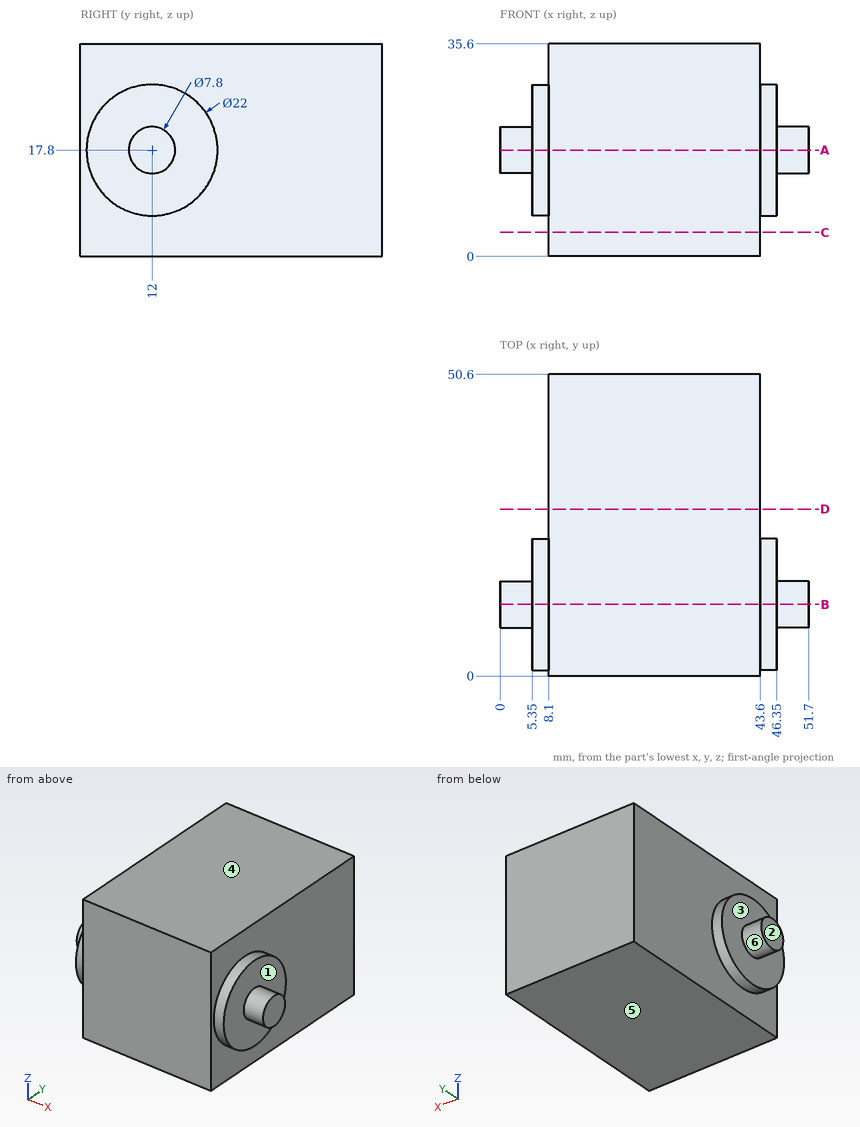
The figure shows three views and two pictorial views of one solid part (mm, origin at its lowest corner). Answer the questions. A direction names the side the tool comes from. Give positions to 0.01 mm unless a question says otherwise; leave off trailing zeros. Loops run counter-clockwise (first coordinate to the right, second up) from the corner with the lowest first, then second, coordinate; pieces in that order, holes last. Notation, with made-up numbers: (-3, 63) -> (56, 63) arc R28 ccw to (56, 85) -> close; hole circle Ø2 at (44, 25). An arc over 180 degrees is marked (long way). Put each result on its own line as item: value. Start each with the question number.
Item 1: Which of the six approach directions +Z, -Z, +X, -X, +Y, -Y give full straight-line access (tool end or side, diameter ignored) to the marked faces 1 and 2?
Item 2: Find the intervals of material crossed by L1, parallel to X at y = 46, z = 6; L2, parallel to X at y = 11, z = 9.5, in increasing order. Write a range as [from, to].
Item 3: The mould has two halves that part along Z. Classify the marked faces 3, 4, 5 and 6: released by +Z, released by -Z, zero draft, split by the parting line, or undercut.
Item 4: The part is cut by section C-C (z = 4). Give the vertices of the cut face in (x, y).
Item 5: The part is cut by section D-D (y = 28). Give the vertices of the cut face in (x, z).
Item 6: The part is cut by section A-A (z = 17.8). Give the vertices of the cut face in (x, y).
Item 7: The part is cut by section B-B (y = 12). Give the vertices of the cut face in (x, z).
Item 8: Each of these flat-tipped pins is pushed along its axis until it touches: P1, Ø2, axis at x = 38, z = 17.5, coming from the -Y side; P2, Ø1.5, axis at y = 35.5, z = 30, coming from the +X side; P3, Ø10, axis at y = 6.5, z = 27.5, coming from the -X side. Where does it stop, or does it pass through?
Answers below:
1. face 1: +X
1. face 2: +Z, -Z, -X, +Y, -Y
2. L1: [8.1, 43.6]
2. L2: [5.35, 46.35]
3. face 3: zero draft
3. face 4: released by +Z
3. face 5: released by -Z
3. face 6: split by the parting line
4. outline: (8.1, 0) -> (43.6, 0) -> (43.6, 50.6) -> (8.1, 50.6) -> close
5. outline: (8.1, 0) -> (43.6, 0) -> (43.6, 35.6) -> (8.1, 35.6) -> close
6. outline: (0, 8.1) -> (5.35, 8.1) -> (5.35, 1) -> (8.1, 1) -> (8.1, 0) -> (43.6, 0) -> (43.6, 1) -> (46.35, 1) -> (46.35, 8.1) -> (51.7, 8.1) -> (51.7, 15.9) -> (46.35, 15.9) -> (46.35, 23) -> (43.6, 23) -> (43.6, 50.6) -> (8.1, 50.6) -> (8.1, 23) -> (5.35, 23) -> (5.35, 15.9) -> (0, 15.9) -> close
7. outline: (0, 13.9) -> (5.35, 13.9) -> (5.35, 6.8) -> (8.1, 6.8) -> (8.1, 0) -> (43.6, 0) -> (43.6, 6.8) -> (46.35, 6.8) -> (46.35, 13.9) -> (51.7, 13.9) -> (51.7, 21.7) -> (46.35, 21.7) -> (46.35, 28.8) -> (43.6, 28.8) -> (43.6, 35.6) -> (8.1, 35.6) -> (8.1, 28.8) -> (5.35, 28.8) -> (5.35, 21.7) -> (0, 21.7) -> close
8. P1: y = 0
8. P2: x = 43.6
8. P3: x = 5.35
